Autodesk Inventor part; units mm, degrees
ref_plane "YZ Plane" through (0, 0, 0) normal (1, 0, 0) x (0, 1, 0)
ref_plane "XZ Plane" through (0, 0, 0) normal (0, 1, 0) x (-1, 0, 0)
ref_plane "XY Plane" through (0, 0, 0) normal (0, 0, 1) x (1, 0, 0)
sketch "Boceto1" plane through (0, 0, 0) normal (1, 0, 0) x (0, 1, 0)
  line L0 (0, 0) -> (20, 0)
  line L1 (20, 0) -> (20, -1)
  line L2 (20, -1) -> (0, -1)
  line L3 (0, -1) -> (0, 0)
  line L4 (0, 0) -> (1, 0)
  line L5 (1, 0) -> (1, -20)
  line L6 (1, -20) -> (0, -20)
  line L7 (0, -20) -> (0, 0)
  point P0 (1, -1)
  dimension "d0" = 20
  dimension "d1" = 20
  dimension "d2" = 1
  dimension "d3" = 1
extrude "Extrusión1" add sketch "Boceto1" along normal blind 200
sketch "Boceto3" plane through (0, 1, -1) normal (0, 1, 0) x (1, 0, 0)
  circle A0 centre (194.35, 3) radius 1.5
  circle A1 centre (163.35, 3) radius 1.5
  line L0 (0, 19) -> (200, 19)
  line L1 (200, 19) -> (200, 0)
  line L2 (0, 0) -> (200, 0)
  point P0 (0, -1)
  dimension "d14" = 3
  dimension "d15" = 3
  dimension "d18" = 5.65
  dimension "d19" = 31
  dimension "d40" = 3
  dimension "d41" = 3
extrude "Extrusión3" cut sketch "Boceto3" against normal through all
sketch "Boceto4" plane through (0, 0, 0) normal (0, 0, 1) x (1, 0, 0)
  circle A0 centre (60.7, 11) radius 2.5
  line L0 (200, 20) -> (200, 0)
  circle A1 centre (93.2, 11) radius 2.5
  line L1 (0, 20) -> (200, 20)
  line L2 (0, 20) -> (0, 0)
  circle A2 centre (141.7, 11) radius 2.5
  dimension "d24" = 9
  dimension "d25" = 9
  dimension "d28" = 5
  dimension "d29" = 5
  dimension "d42" = 60.7
  dimension "d43" = 32.5
  dimension "d44" = 5
  dimension "d45" = 9
  dimension "d46" = 48.5
extrude "Extrusión4" cut sketch "Boceto4" against normal through all
sketch "Boceto5" plane through (0, 1, -1) normal (0, 1, 0) x (1, 0, 0)
  circle A0 centre (65.7, 10) radius 2.5
  line L0 (0, 19) -> (0, 0)
  circle A1 centre (130.7, 10) radius 2.5
  line L1 (0, 19) -> (200, 19)
  point P0 (0, -1)
  dimension "d30" = 5
  dimension "d32" = 65.7
  dimension "d33" = 5
  dimension "d39" = 65
  dimension "d62" = 9
  dimension "d63" = 9
extrude "Extrusión5" cut sketch "Boceto5" against normal through all
sketch "Boceto6" plane through (0, 1, -1) normal (0, 0, -1) x (-1, 0, 0)
  circle A0 centre (-190, 6.5) radius 1.5
  circle A1 centre (-168, 6.5) radius 1.5
  line L0 (-200, 0) -> (-200, 19)
  line L1 (0, 0) -> (-200, 0)
  point P0 (0, -1)
  dimension "d47" = 3
  dimension "d48" = 3
  dimension "d49" = 10
  dimension "d51" = 6.5
  dimension "d52" = 6.5
  dimension "d55" = 32
extrude "Extrusión6" cut sketch "Boceto6" against normal through all
sketch "Boceto7" plane through (0, 1, -1) normal (0, 1, 0) x (1, 0, 0)
  circle A0 centre (175.7, 14) radius 1.5
  line L0 (0, 0) -> (200, 0)
  line L1 (200, 19) -> (200, 0)
  line L2 (0, 19) -> (200, 19)
  point P0 (0, -1)
  dimension "d57" = 24.3
  dimension "d60" = 3
  dimension "d61" = 5
extrude "Extrusión7" cut sketch "Boceto7" against normal through all
equation "\"d1\" = d0"
equation "\"d3\" = d2"
equation "\"d15\" = d14"
equation "\"d41\" = d40"
equation "\"d24\" = d25"
equation "\"d29\" = d28"
equation "\"d44\" = d29"
equation "\"d45\" = d25"
equation "\"d33\" = d30"
equation "\"d63\" = d62"
equation "\"d48\" = d47"
equation "\"d52\" = d51"
properties part number "Angulo 2020x450" material "Madera (cerezo)"
Check sheet for the modelled part. Datum: model origin and axes. Units: mm. A direction names the side the tool comes from. Round coordinates to 2 decimals unless told otherwise and drop trailing zeros. Write each loop counter-clockwise with the first axis right and the second up, starting at its lowest first coordinate (ties: lowest second). Pieces come first, ordered by that corner, then holes. Notation, with made-up numbers: M -33.5,-3 L -29.5,-3 A32 cw -29.5,30 Z; hole C 40.5,71 d3. An arc over 180 degrees is marked long. Write item = value, one per line. Start each with the question number.
1. Section check C-C, the plane y = 17.5. Record the cut outline in (x, z), then the cut area to 3 significant figures.
2. Tool access check on faces 1 (the cylindrical face through (58.2, 11.1, -0.5)), 2 (the flat face through (99, 1, -10)). Record the directions out of +Z, -Z, +X, -X, +Y, -Y that give a thin tool (end or side, any length) a straight path to the whole face; none if there is none.
3. Section check B-B, the plane x = 40. Record the cut outline in (y, z).
4. Release check for a two-part mould opening along X. For faces 3 (the flat face through (99, 11, -1)), 4 (the flat face through (200, 5.5, -0.3)), 5 (the cylindrical face through (94.35, 8.78, -0.49)), 6 (the flat face through (0, 5.5, -0.3)) record: pulls with the +X half, pulls with the -X half, needs draft (parallel to the pull), parting line crosses it, or undercut.
5. Section check A-A, the plane x = 93.2. Record the cut outline in (y, z).
6. Scan lines: line 1 (X direction, y = 0.55, z = -11); line 2 (X direction, y = 0.3, z = -4); line 3 (Z direction, x = 163.35, y = 0.7). Record each from-to range of solid material in increasing order. Write a range as [from, to].
7. Gauge pin test, flat ends, axial feed: pin 1 (6 mm diameter, centred on x = 130.7, z = -11, fed in from +Y); pin 2 (8 mm diameter, centred on x = 117, z = -4, fed in from +Y); pin 3 (8 mm diameter, centred on x = 93.2, y = 11, fed in from -Z). Record the tip position at first contact, or that the pin passes through.
Results found:
q1.outline = M 0,-1 L 200,-1 L 200,0 L 0,0 Z
q1.area = 200 mm^2
q2.face_1 = +Z, -Z
q2.face_2 = -Z, +X, -X, +Y
q3.outline = M 0,-20 L 1,-20 L 1,-1 L 20,-1 L 20,0 L 0,0 Z
q4.face_3 = needs draft
q4.face_4 = pulls with the +X half
q4.face_5 = undercut
q4.face_6 = pulls with the -X half
q5.outline = M 0,-20 L 1,-20 L 1,-1 L 8.5,-1 L 8.5,0 L 0,0 Z; M 13.5,-1 L 20,-1 L 20,0 L 13.5,0 Z
q6.line_1 = [0, 63.2], [68.2, 128.2], [133.2, 200]
q6.line_2 = [0, 161.85], [164.85, 192.85], [195.85, 200]
q6.line_3 = [-20, -5.5], [-2.5, 0]
q7.pin_1 = 1
q7.pin_2 = 20
q7.pin_3 = -1
